Source: CAD feature listing. Evaluate the final solid. Frame: model axes, mm. A direction names the side the tool comes from. Give positions to 0.01 mm unless a question says otherwise; leave off trailing zeros. Loops run counter-clockwise (first coordinate to the right, second up) from the corner with the lowest first, then second, coordinate; pieces in that order, holes last. Notation, with made-up numbers: M 43.25,-29 L 91.25,-29 A16 cw 91.25,-1 Z; hole C 6.5,-5.5 d4. An arc over 180 degrees is marked long. Answer in a Markdown table with one row per item.
Autodesk Fusion 360 part; units mm, degrees
box "BoxPrimitive1" add length 3.5 width 10 height 7 placed x (0, 1, 0) y (-1, 0, 0) z (0, 0, 1) at (10, 0, 0)
sketch "Sketch2" plane through (0, 0, 7) normal (0, 0, 1) x (-1, 0, 0)
  line L0 (-10, -3.5) -> (0, -3.5)
  line L1 (0, -3.5) -> (0, 0)
  line L2 (0, 0) -> (-10, 0)
  line L3 (-10, 0) -> (-10, -3.5)
  line L4 (-5, -3.5) -> (-5, -1.75)
  line L5 (-6.4, -0.35) -> (-3.6, -0.35)
  line L6 (-3.6, -0.35) -> (-3.6, -3.15)
  line L7 (-3.6, -3.15) -> (-6.4, -3.15)
  line L8 (-6.4, -3.15) -> (-6.4, -0.35)
  line L9 (-6.4, -0.35) -> (-3.6, -3.15) construction
  line L10 (-3.6, -0.35) -> (-6.4, -3.15) construction
  point P0 (-5, -1.75)
  dimension "d6" = 1.75
  dimension "d7" = 2.8
  dimension "d8" = 2.8
extrude "Extrude1" cut sketch "Sketch2" against normal blind 3.5
sketch "Sketch3" plane through (0, 0, 0) normal (0, 0, -1) x (1, 0, 0)
  line L0 (0, -3.5) -> (10, -3.5)
  line L1 (10, -3.5) -> (10, 0)
  line L2 (10, 0) -> (0, 0)
  line L3 (0, 0) -> (0, -3.5)
  line L4 (5.875, -2.625) -> (4.125, -2.625)
  line L5 (4.125, -2.625) -> (4.125, -0.875)
  line L6 (4.125, -0.875) -> (5.875, -0.875)
  line L7 (5.875, -0.875) -> (5.875, -2.625)
  line L8 (5.875, -2.625) -> (4.125, -0.875) construction
  line L9 (4.125, -2.625) -> (5.875, -0.875) construction
  line L10 (4.125, -0.875) -> (5.875, -0.875)
  line L11 (5.875, -0.875) -> (5.875, 0)
  line L12 (5.875, 0) -> (4.125, 0)
  line L13 (4.125, 0) -> (4.125, -0.875)
  point P0 (5, -1.75)
  point P1 (5, -1.75)
  dimension "d11" = 1.75
  dimension "d12" = 1.75
  dimension "d17" = 1.75
extrude "Extrude2" cut sketch "Sketch3" against normal blind 3.5 contours L4 L5 L6 L7 L10
extrude "Extrude3" add sketch "Sketch2" along normal blind 1 contours L5 L6 L7 L8
extrude "Extrude4" cut sketch "Sketch3" against normal blind 3.5 contours L2 L6 L10 L11 L12 L13
extrude "Extrude5" add 1 faces at (8.8, 1.2833, 3.5) along direction (0, 0, 1) blind 0.7
sketch "Sketch4" plane through (0, 0.35, 0) normal (0, -1, 0) x (1, 0, 0)
  line L0 (5.875, 4.2) -> (6.4, 4.2)
  line L1 (6.4, 4.2) -> (6.4, 8)
  line L2 (6.4, 8) -> (3.6, 8)
  line L3 (3.6, 8) -> (3.6, 4.2)
  line L4 (3.6, 4.2) -> (4.125, 4.2)
  line L5 (4.125, 4.2) -> (4.125, 3.5)
  line L6 (4.125, 3.5) -> (5.875, 3.5)
  line L7 (5.875, 3.5) -> (5.875, 4.2)
  line L8 (4.125, 3.5) -> (5.875, 3.5)
  line L9 (5.875, 3.5) -> (5.875, 4.2)
  line L10 (5.875, 4.2) -> (4.125, 4.2)
  line L11 (4.125, 4.2) -> (4.125, 3.5)
extrude "Extrude6" add sketch "Sketch4" along normal blind 0.35 contours L5 L6 L7 L8 L9 L10 L11
extrude "Extrude7" cut 1 faces at (5.4667, 1.2833, 8) along direction (0, 0, -1) blind 0.5
Q1. Contact query for flat-ended pins moving along their axis: pin 1 Ø1.4 at (y, z) = (2, 5) entering from +X; pin 2 Ø2 at (x, z) = (6.5, 6.5) entering from +Y; pin 3 Ø1.4 at (x, z) = (5.5, 6) entering from -Y. Output: stop coordinate, or through.
Values follow:
| item | result |
|---|---|
| pin 1 | x = 6.4 |
| pin 2 | y = 3.15 |
| pin 3 | y = 0.35 |
Q2. Ray query, probe 1 along X at (y, z) = (0.65, 3.25) (3 decimals); probe 2 along Z at (x, y) = (1.75, 2.85); probe 3 along Y at (x, z) = (4, 7). Return the intervals inside material, ascending. Write a range as from..to.
Values follow:
| item | result |
|---|---|
| probe 1 | 0..4.125, 5.875..10 |
| probe 2 | 0..4.2 |
| probe 3 | 0.35..3.15 |
Q3. Section query D-D (x = 7.75). Output: boundary loops of the cut face in (y, z), plus the area to 3 significant figures.
Values follow:
| item | result |
|---|---|
| outline | M 0,0 L 3.5,0 L 3.5,4.2 L 0,4.2 Z |
| area | 14.7 mm^2 |
Q4. Section query C-C (z = 1.25). Output: boundary loops of the cut face in (x, y) (3 decimals), plus the area to 3 significant figures.
Values follow:
| item | result |
|---|---|
| outline | M 0,0 L 4.125,0 L 4.125,2.625 L 5.875,2.625 L 5.875,0 L 10,0 L 10,3.5 L 0,3.5 Z |
| area | 30.4 mm^2 |
Q5. Section query A-A (x = 4.25). Output: boundary loops of the cut face in (y, z) (3 decimals), plus the area to 3 significant figures.
Values follow:
| item | result |
|---|---|
| outline | M 0,3.5 L 2.625,3.5 L 2.625,0 L 3.5,0 L 3.5,4.2 L 3.15,4.2 L 3.15,7.5 L 0.35,7.5 L 0.35,4.2 L 0,4.2 Z |
| area | 14.8 mm^2 |
Q6. Reachability of faces 4 (the flat face through (5, 1, 3.5)), 5 (the flat face through (5, 3.15, 6)), 6 (the flat face through (6.4, 2, 6)), 7 (the flat face through (5, 0.35, 6)), 8 (the flat face through (3.6, 2, 6)) from +Z, -Z, +X, -X, +Y, -Y: full face, straight path, thin tool, end or side. Return the list, or none.
Values follow:
| item | result |
|---|---|
| face 4 | -Z, -Y |
| face 5 | +Z, +X, -X, +Y |
| face 6 | +Z, +X, +Y, -Y |
| face 7 | +Z, +X, -X, -Y |
| face 8 | +Z, -X, +Y, -Y |
Q7. Section query B-B (y = 0.55). Output: boundary loops of the cut face in (x, z) (3 decimals), plus the area to 3 significant figures.
Values follow:
| item | result |
|---|---|
| outline | M 0,0 L 4.125,0 L 4.125,3.5 L 5.875,3.5 L 5.875,0 L 10,0 L 10,4.2 L 6.4,4.2 L 6.4,7.5 L 3.6,7.5 L 3.6,4.2 L 0,4.2 Z |
| area | 45.1 mm^2 |
Q8. Mould query, pull axis X, two halves, no side actions, for faces 1 (the flat face through (5, 2.625, 2)), 2 (the flat face through (3.8, 1.7, 0)), 3 (the flat face through (10, 2, 2)). Classes: +X half, -X half, draft (parallel to the pull), parting line (faces both ways), or undercut.
Values follow:
| item | result |
|---|---|
| face 1 | undercut |
| face 2 | draft |
| face 3 | +X half |
